```python
from build123d import *

# Parameters (mm, degrees)
F1_DEPTH = 3
F2_R     = 5
F3_D     = 2.5


with BuildPart() as f1:
    # F0 (on Top) → F1 (new body)
    with BuildSketch(Plane.XY):
        with BuildLine():
            ThreePointArc((1.4295431963, 7.3625), (2.5776568419, 8.4651758389), (3, 10))
            ThreePointArc((3, 10), (-1.5348241611, 12.5776568419), (-1.4295431963, 7.3625))
            ThreePointArc((-1.4295431963, 7.3625), (0, 7.5), (1.4295431963, 7.3625))
        make_face()
        with BuildLine():
            ThreePointArc((1.4295431963, -7.3625), (0, -7), (-1.4295431963, -7.3625))
            ThreePointArc((-1.4295431963, -7.3625), (0, -7.5), (1.4295431963, -7.3625))
        make_face()
        with BuildLine():
            ThreePointArc((1.4295431963, 7.3625), (0, 7), (-1.4295431963, 7.3625))
            ThreePointArc((-1.4295431963, 7.3625), (-7.5, 0), (-1.4295431963, -7.3625))
            ThreePointArc((-1.4295431963, -7.3625), (0, -7), (1.4295431963, -7.3625))
            ThreePointArc((1.4295431963, -7.3625), (5.7866905037, -4.7711857032), (7.5, 0))
            ThreePointArc((7.5, 0), (5.7866905037, 4.7711857032), (1.4295431963, 7.3625))
        make_face()
        with BuildLine():
            ThreePointArc((1.4295431963, 7.3625), (0, 7.5), (-1.4295431963, 7.3625))
            ThreePointArc((-1.4295431963, 7.3625), (0, 7), (1.4295431963, 7.3625))
        make_face()
        with BuildLine():
            ThreePointArc((1.4295431963, -7.3625), (0, -7.5), (-1.4295431963, -7.3625))
            ThreePointArc((-1.4295431963, -7.3625), (-1.5348241611, -12.5776568419), (3, -10))
            ThreePointArc((3, -10), (2.5776568419, -8.4651758389), (1.4295431963, -7.3625))
        make_face()
    extrude(amount=F1_DEPTH)

    # F2
    f2_edges = [f1.edges().sort_by_distance(p)[0] for p in [
        (-1.429543, -7.3625, 1.5),
        (1.429543, -7.3625, 1.5),
        (-1.429543, 7.3625, 1.5),
        (1.429543, 7.3625, 1.5),
    ]]
    fillet(f2_edges, radius=F2_R)

    # F3 (through all)
    with Locations(Plane(origin=(0, 0, 0), x_dir=(1, 0, 0), z_dir=(0, 0, -1))):
        with Locations((0, 10), (0, -10)):
            Hole(F3_D / 2)


solid = f1.part
```
Work out the finished part from the listing and answer in its coordinate system (mm). Give positions to 0.01 mm unless a question says otherwise; leave off trailing zeros. Write each loop counter-clockwise with the first axis right and the second up, starting at its lowest first coordinate (ties: lowest second). Pieces come first, ordered by that corner, then holes.
(1) The part is cut by section D-D on z = 2. Count the separate pieces of the cut face and the enclosed holes in it, plus the area to 3 significant figures.
Final values:
separate pieces: 1
enclosed holes: 2
area: 232 mm2
(2) The part is cut by section A-A on x = 0. Write down the section's boundary in (y, z), plus the area to 3 significant figures.
Final values:
outline: (-13, 0) - (-11.25, 0) - (-11.25, 3) - (-13, 3) - close; (-8.75, 0) - (8.75, 0) - (8.75, 3) - (-8.75, 3) - close; (11.25, 0) - (13, 0) - (13, 3) - (11.25, 3) - close
area: 63.0 mm2
(3) Straight lines are drawn through the part: line 1 (Y direction, x = 0, z = 2.35); line 2 (X direction, y = -10, z = 2.1); line 3 (X direction, y = -9.25, z = 1.85). For each, find the intervals that lie inside material, in ascending order.
Final values:
line 1: y = -13 to -11.25, -8.75 to 8.75, 11.25 to 13
line 2: x = -3 to -1.25, 1.25 to 3
line 3: x = -3 to -1, 1 to 3
(4) The part is cut by section B-B on y = -10.25. Write down the section's boundary in (x, z).
Final values:
outline: (-2.99, 0) - (-1.22, 0) - (-1.22, 3) - (-2.99, 3) - close; (1.22, 0) - (2.99, 0) - (2.99, 3) - (1.22, 3) - close
(5) A flat-ended cylindrical pin translates along its axis: pin 1 Ø2 at (x, y) = (0, 10) entering from +Z. Find the tip coordinate at first contact, or state that the pin passes through.
Final values:
pin 1: passes through
(6) The part is cut by section C-C on y = 2. Write down the section's boundary in (x, z).
Final values:
outline: (-7.23, 0) - (7.23, 0) - (7.23, 3) - (-7.23, 3) - close
(7) The mould has two halves that part along Y. Classify faces 1 (the cylindrical face through (-0.672, 8.946, 1.521)), 2 (the cylindrical face through (7.5, -0.1, 1.5)), 3 (the flat face through (0, 0, 3)), 4 (the cylindrical face through (0.16, -11.24, 1.52)): pulls with the +Y half, pulls with the -Y half, needs draft (parallel to the pull), parting line crosses it, or undercut.
Final values:
face 1: undercut
face 2: parting line crosses it
face 3: needs draft
face 4: undercut
